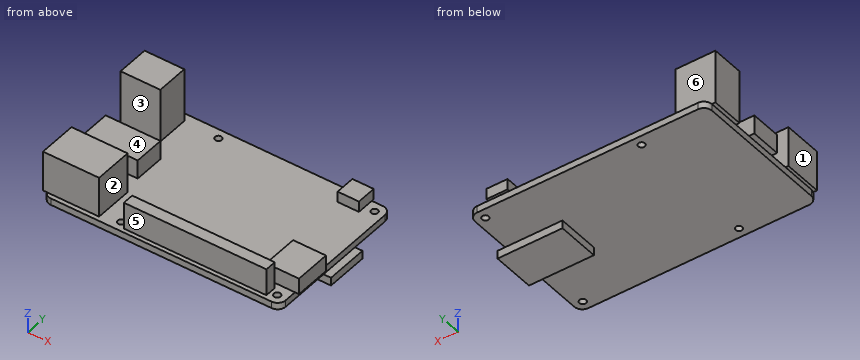
from build123d import *

# Parameters (mm, degrees)
SKETCH_1_W      = 88
SKETCH_1_H      = 56
SKETCH_1_R      = 1.25
EXTRUDE_1_DEPTH = 2.5
SKETCH_3_W      = 14.749474834
SKETCH_3_H      = 12.067752137
EXTRUDE_2_DEPTH = 20
SKETCH_4_W      = 20.823165918
SKETCH_4_H      = 14.358457545
EXTRUDE_3_DEPTH = 15
SKETCH_5_W      = 20.346818985
SKETCH_5_H      = 11.432326386
EXTRUDE_4_DEPTH = 7
SKETCH_6_W      = 52.92270657
SKETCH_6_H      = 4.181716452
EXTRUDE_5_DEPTH = 10
SKETCH_7_W      = 12.202385712
SKETCH_7_H      = 13.573440286
EXTRUDE_6_DEPTH = 6
SKETCH_8_W      = 24.111474105
SKETCH_8_H      = 15.818799485
EXTRUDE_7_DEPTH = 3
SKETCH_9_W      = 7.916095885
SKETCH_9_H      = 7.421339892
EXTRUDE_8_DEPTH = 4
FILLET_1_R      = 3


with BuildPart() as part:
    # 草图1 → 凸台-拉伸1 (new body)
    with BuildSketch(Plane.XY):
        Rectangle(SKETCH_1_W, SKETCH_1_H)
        with Locations((-17.5, 24.5)):
            Circle(SKETCH_1_R, mode=Mode.SUBTRACT)
        with Locations((40.5, 24.5)):
            Circle(SKETCH_1_R, mode=Mode.SUBTRACT)
        with Locations((40.5, -24.5)):
            Circle(SKETCH_1_R, mode=Mode.SUBTRACT)
        with Locations((-17.5, -24.5)):
            Circle(SKETCH_1_R, mode=Mode.SUBTRACT)
    extrude(amount=EXTRUDE_1_DEPTH)

    # 草图3 → 凸台-拉伸2 (add)
    with BuildSketch(Plane.XY.offset(2.5)):
        with Locations((-37.946376164, 19.006709616)):
            Rectangle(SKETCH_3_W, SKETCH_3_H)
    extrude(amount=EXTRUDE_2_DEPTH)

    # 草图4 → 凸台-拉伸3 (add)
    with BuildSketch(Plane.XY.offset(2.5)):
        with Locations((-34.685337702, -19.189976435)):
            Rectangle(SKETCH_4_W, SKETCH_4_H)
    extrude(amount=EXTRUDE_3_DEPTH)

    # 草图5 → 凸台-拉伸4 (add)
    with BuildSketch(Plane.XY.offset(2.5)):
        with Locations((-35.808155473, 0.646470837)):
            Rectangle(SKETCH_5_W, SKETCH_5_H)
    extrude(amount=EXTRUDE_4_DEPTH)

    # 草图6 → 凸台-拉伸5 (add)
    with BuildSketch(Plane.XY.offset(2.5)):
        with Locations((11.485814144, -24.404771423)):
            Rectangle(SKETCH_6_W, SKETCH_6_H)
    extrude(amount=EXTRUDE_5_DEPTH)

    # 草图7 → 凸台-拉伸6 (add)
    with BuildSketch(Plane.XY.offset(2.5)):
        with Locations((39.386774732, -13.539163922)):
            Rectangle(SKETCH_7_W, SKETCH_7_H)
    extrude(amount=EXTRUDE_6_DEPTH)

    # 草图8 → 凸台-拉伸7 (add)
    with BuildSketch(Plane(origin=(0, 0, 0), x_dir=(-1, 0, 0), z_dir=(0, 0, -1))):
        with Locations((-34.735744668, 1.951217558)):
            Rectangle(SKETCH_8_W, SKETCH_8_H)
    extrude(amount=EXTRUDE_7_DEPTH)

    # 草图9 → 凸台-拉伸8 (add)
    with BuildSketch(Plane.XY.offset(2.5)):
        with Locations((32.917495051, 25.232555635)):
            Rectangle(SKETCH_9_W, SKETCH_9_H)
    extrude(amount=EXTRUDE_8_DEPTH)

    # 圆角1
    # the kernel refuses this fillet: 3 mm, written as the material it takes off along each edge
    with BuildSketch(Plane(origin=(44, -28, -7.5), x_dir=(-1, 0, 0), z_dir=(0, 0, 1)), Plane(origin=(44, 28, -7.5), x_dir=(0, -1, 0), z_dir=(0, 0, 1))) as fillet_1_piece_1:
        with BuildLine():
            CenterArc((FILLET_1_R, -FILLET_1_R), FILLET_1_R, 90, 90)
            Line((0, -FILLET_1_R), (0, 0))
            Line((0, 0), (FILLET_1_R, 0))
        make_face()
    extrude(amount=17.5, mode=Mode.SUBTRACT)
    with BuildSketch(Plane(origin=(-44, -28, -7.5), x_dir=(1, 0, 0), z_dir=(0, 0, 1)), Plane(origin=(-44, 28, -7.5), x_dir=(0, -1, 0), z_dir=(0, 0, 1))) as fillet_1_piece_2:
        with BuildLine():
            CenterArc((FILLET_1_R, FILLET_1_R), FILLET_1_R, 180, 90)
            Line((0, FILLET_1_R), (0, 0))
            Line((0, 0), (FILLET_1_R, 0))
        make_face()
    extrude(amount=10, mode=Mode.SUBTRACT)


solid = part.part
Work out the finished part from the listing and answer in its coordinate system (mm). Face numbers are marked on the shaded views. A direction names the side the tool comes from. Give positions to 0.01 mm unless a question says otherwise; leave off trailing zeros. Order: outer loops, then holes, each group sorted by start corner. A loop starts at its lowest first (then second) coordinate and runs counter-clockwise, first axis right, second up. Notation, with made-up numbers: (53.25, -34) -> (99.25, -34) arc R20 ccw to (99.25, -22) -> close; hole circle Ø7 at (74.5, -2). An arc over 180 degrees is marked (long way). Answer as a JSON object with one key per item and string values. Group by question number.
1. Section D-D on z = 4.75 is taken. Determine the outline of the cut face in (x, y).
2. Consider line 1 along Y through (x, z) = (-17.5, 0.95); line 2 along Z through (x, y) = (-8.5, 17.5); line 3 along Z through (x, y) = (-35, -22). Determine where each line is inside the solid, lowest interval first. Write a range as [from, to].
3. Flat-ended cylindrical pins translate along their axes: pin 1 Ø3 at (y, z) = (27, 3.5) entering from -X; pin 2 Ø4.5 at (x, z) = (-35.5, 9.5) entering from -Y; pin 3 Ø2 at (x, z) = (-11.5, 12.5) entering from -Y. Find the tip coordinate at first contact, or state that the pin passes through.
4. A tool of negligible diameter and unlimited length cuts with its end or side. For the marked faces 4, 5 and 6, from which of +Z, -Z, +X, -X, +Y, -Y can it reach the whole face along a straight path? Write none if from no direction.
5. Section A-A on x = -17.5 is taken. Determine the outline of the cut face in (y, z), plus the area to 4 significant figures.
6. The mould has two halves that part along X. Classify the marked faces 1, 2 and 3: released by +X, released by -X, zero draft, split by the parting line, or undercut.
7. Section B-B on z = 15 is taken. Determine the outline of the cut face in (x, y).
8. Section C-C on y = 16 is taken. Determine the outline of the cut face in (x, z).
Result sheet:
{
 "1": {"outline": "(-45.98, -5.07) -> (-25.63, -5.07) -> (-25.63, 6.36) -> (-45.98, 6.36) -> close; (-45.32, 12.97) -> (-30.57, 12.97) -> (-30.57, 25.04) -> (-45.32, 25.04) -> close; (-45.1, -26.37) -> (-24.27, -26.37) -> (-24.27, -12.01) -> (-45.1, -12.01) -> close; (-14.98, -26.5) -> (37.95, -26.5) -> (37.95, -22.31) -> (-14.98, -22.31) -> close; (28.96, 21.52) -> (36.88, 21.52) -> (36.88, 28.94) -> (28.96, 28.94) -> close; (33.29, -20.33) -> (45.49, -20.33) -> (45.49, -6.75) -> (33.29, -6.75) -> close"},
 "2": {"line 1": "y = [-28, -25.75], [-23.25, 23.25], [25.75, 28]", "line 2": "z = [0, 2.5]", "line 3": "z = [0, 17.5]"},
 "3": {"pin 1": "stops at x = -43.87", "pin 2": "stops at y = -26.37", "pin 3": "stops at y = -26.5"},
 "4": {"face 4": "+Z, +X, -X", "face 5": "+Z, +X, -X, -Y", "face 6": "+Z, -X, +Y"},
 "5": {"outline": "(-28, 0) -> (-25.75, 0) -> (-25.75, 2.5) -> (-28, 2.5) -> close; (-23.25, 0) -> (23.25, 0) -> (23.25, 2.5) -> (-23.25, 2.5) -> close; (25.75, 0) -> (28, 0) -> (28, 2.5) -> (25.75, 2.5) -> close", "area": "127.5 mm^2"},
 "6": {"face 1": "released by -X", "face 2": "undercut", "face 3": "zero draft"},
 "7": {"outline": "(-45.32, 12.97) -> (-30.57, 12.97) -> (-30.57, 25.04) -> (-45.32, 25.04) -> close; (-45.1, -26.37) -> (-24.27, -26.37) -> (-24.27, -12.01) -> (-45.1, -12.01) -> close"},
 "8": {"outline": "(-45.32, 2.5) -> (-44, 2.5) -> (-44, 0) -> (44, 0) -> (44, 2.5) -> (-30.57, 2.5) -> (-30.57, 22.5) -> (-45.32, 22.5) -> close"}
}
